```python
from build123d import *

# Parameters (mm, degrees)
SKETCH2_W           = 600
SKETCH2_H           = 530
SKETCH2_W_2         = 570
SKETCH2_H_2         = 500
BASE_EXTRUDE_DEPTH  = 50
SKETCH3_W           = 600
SKETCH3_H           = 580
BOSS_EXTRUDE2_DEPTH = 15
SKETCH4_W           = 600
SKETCH4_H           = 580
SKETCH4_W_2         = 570
SKETCH4_H_2         = 550
BOSS_EXTRUDE3_DEPTH = 800
CUT_EXTRUDE1_REACH  = 1203.926
SKETCH5_W           = 420
SKETCH5_H           = 635
SKETCH6_R           = 11.180339887
SKETCH6_R_2         = 27.5
CUT_EXTRUDE2_DEPTH  = 1195.759390003


with BuildPart() as part:
    # Sketch2 → Base-Extrude (new body)
    with BuildSketch(Plane.XY):
        with Locations((300, -265)):
            Rectangle(SKETCH2_W, SKETCH2_H)
        with Locations((300, -265)):
            Rectangle(SKETCH2_W_2, SKETCH2_H_2, mode=Mode.SUBTRACT)
    extrude(amount=BASE_EXTRUDE_DEPTH)

    # Sketch3 → Boss-Extrude2 (add)
    with BuildSketch(Plane.XY.offset(50)):
        with Locations((300, -290)):
            Rectangle(SKETCH3_W, SKETCH3_H)
    extrude(amount=BOSS_EXTRUDE2_DEPTH)

    # Sketch4 → Boss-Extrude3 (add)
    with BuildSketch(Plane.XY.offset(65)):
        with Locations((300, -290)):
            Rectangle(SKETCH4_W, SKETCH4_H)
        with Locations((300, -290)):
            Rectangle(SKETCH4_W_2, SKETCH4_H_2, mode=Mode.SUBTRACT)
    extrude(amount=BOSS_EXTRUDE3_DEPTH)

    # Sketch5 → Cut-Extrude1 (cut, up to next)
    with BuildSketch(Plane.XZ.offset(580), mode=Mode.PRIVATE) as cut_extrude1_sk1:
        with Locations((300, 457.5)):
            Rectangle(SKETCH5_W, SKETCH5_H)
    cut_extrude1_tool1 = extrude(cut_extrude1_sk1.sketch, amount=-CUT_EXTRUDE1_REACH, mode=Mode.PRIVATE) & part.part
    add(cut_extrude1_tool1.solids().sort_by_distance((300, -580, 457.5))[0], mode=Mode.SUBTRACT)

    # Sketch6 → Cut-Extrude2 (cut, through all)
    with BuildSketch(Plane.XZ.offset(15)):
        with Locations(Location((355, 565, 0), (0, 0, 270))):
            Circle(SKETCH6_R)
        with Locations(Location((255, 565, 0), (0, 0, 270))):
            Circle(SKETCH6_R)
        with Locations(Location((300, 595, 0), (0, 0, 270))):
            Circle(SKETCH6_R_2)
    extrude(amount=-CUT_EXTRUDE2_DEPTH, mode=Mode.SUBTRACT)


solid = part.part
```
Model file for the job. Use its own axes, mm. A direction names the side the tool comes from. Give positions to 0.01 mm unless a question says otherwise; leave off trailing zeros. Loops run counter-clockwise (first coordinate to the right, second up) from the corner with the lowest first, then second, coordinate; pieces in that order, holes last. Notation, with made-up numbers: (35, 41) -> (89, 41) arc R8 cw to (89, 49) -> close; hole circle Ø8 at (83.5, -7). An arc over 180 degrees is marked (long way). Use CSV: the item, a comma, the result in double quotes. Start each with the question number.
1) Mould opens along X. For faces 4 (the flat face through (0, -294, 426)), 5 (the flat face through (15, -294, 459)), 6 (the flat face through (276, -519, 0)) say: released by +X, released by -X, zero draft, split by the parting line, or undercut.
2) Slice it at C-C on x = 164.5. Give the cut face in (y, z), plus the area to 3 significant figures.
3) Slice it at B-B on z = 595. Give the cut face in (x, y), plus the area to 3 significant figures.
4) Slice it at D-D on y = -94. Give the cut face in (x, z).
5) Tool access for faces 1 (the flat face through (296, -555, 50)), 2 (the flat face through (585, -268, 25)), 3 (the flat face through (296, -286, 65)): list every direction of +Z, -Z, +X, -X, +Y, -Y with a clear straight run to the whole face (end or side of a thin tool).
6) Wall check: line 1 (X direction, y = -5.25, z = 565); line 2 (Y direction, x = 52, z = 297); line 3 (X direction, y = -6, z = 595). Give the ranges that are in metal, low to high.
7) Slice it at A-A on x = 255. Give the cut face in (y, z), plus the area to 3 significant figures.
8) Flat gauge pins, fed straight in: pin 1 Ø25 at (x, y) = (390.5, -555) entering from -Z; pin 2 Ø6 at (x, y) = (512, -425) entering from +Z; pin 3 Ø6 at (x, z) = (455.5, 306) entering from -Y. Where does each tip first touch, or does it go through?
Computed values:
1,face 4,"released by -X"
1,face 5,"undercut"
1,face 6,"zero draft"
2,outline,"(-580, 50) -> (-530, 50) -> (-530, 0) -> (-515, 0) -> (-515, 50) -> (-15, 50) -> (-15, 0) -> (0, 0) -> (0, 865) -> (-15, 865) -> (-15, 65) -> (-565, 65) -> (-565, 140) -> (-580, 140) -> close; (-580, 775) -> (-565, 775) -> (-565, 865) -> (-580, 865) -> close"
2,area,"24,700 mm^2"
3,outline,"(0, -580) -> (90, -580) -> (90, -565) -> (15, -565) -> (15, -15) -> (272.5, -15) -> (272.5, 0) -> (0, 0) -> close; (327.5, -15) -> (585, -15) -> (585, -565) -> (510, -565) -> (510, -580) -> (600, -580) -> (600, 0) -> (327.5, 0) -> close"
3,area,"27,400 mm^2"
4,outline,"(0, 0) -> (15, 0) -> (15, 50) -> (585, 50) -> (585, 0) -> (600, 0) -> (600, 865) -> (585, 865) -> (585, 65) -> (15, 65) -> (15, 865) -> (0, 865) -> close"
5,face 1,"-Z, +X, -X, -Y"
5,face 2,"-Z"
5,face 3,"+Z"
6,line 1,"x = 0 to 243.82, 266.18 to 343.82, 366.18 to 600"
6,line 2,"y = -580 to -565, -15 to 0"
6,line 3,"x = 0 to 272.5, 327.5 to 600"
7,outline,"(-580, 50) -> (-530, 50) -> (-530, 0) -> (-515, 0) -> (-515, 50) -> (-15, 50) -> (-15, 0) -> (0, 0) -> (0, 553.82) -> (-15, 553.82) -> (-15, 65) -> (-565, 65) -> (-565, 140) -> (-580, 140) -> close; (-580, 775) -> (-565, 775) -> (-565, 865) -> (-580, 865) -> close; (-15, 576.18) -> (0, 576.18) -> (0, 865) -> (-15, 865) -> close"
7,area,"24,300 mm^2"
8,pin 1,"stops at z = 50"
8,pin 2,"stops at z = 65"
8,pin 3,"stops at y = -15"
